Geometry: final body of the model. Coordinates: model frame, mm. Face numbers are marked on the shaded views. A direction names the side the tool comes from. Coordinates: 2 decimals unless noted, no trailing zeros. Order: outer loops, then holes, each group sorted by start corner. A loop starts at its lowest first (then second) coordinate and runs counter-clockwise, first axis right, second up. Notation, with made-up numbers: M 19.25,13 L 35.25,13 A19 ccw 35.25,47 Z; hole C 86.5,88.5 d8. An arc over 180 degrees is marked long. Write item = value, one per line.
from build123d import *

# Parameters (mm, degrees)
SKETCH1_W             = 25
SKETCH1_H             = 60
BOSS_EXTRUDE1_DEPTH   = 5
SKETCH8_W             = 5
SKETCH8_H             = 60
BOSS_EXTRUDE2_DEPTH   = 80
SKETCH9_R             = 2.1
SKETCH9_W             = 20
SKETCH9_H             = 40
CUT_EXTRUDE1_DEPTH    = 5
CUT_EXTRUDE2_REACH    = 7
FILLET1_R             = 2.5
F_3_0MM_DOWEL_HOLE1_D = 3


with BuildPart() as part:
    # Sketch1 → Boss-Extrude1 (new body)
    with BuildSketch(Plane(origin=(0, 0, 0), x_dir=(1, 0, 0), z_dir=(0, 1, 0))):
        Rectangle(SKETCH1_W, SKETCH1_H)
    extrude(amount=BOSS_EXTRUDE1_DEPTH)

    # Sketch8 → Boss-Extrude2 (add)
    with BuildSketch(Plane(origin=(0, 5, 0), x_dir=(1, 0, 0), z_dir=(0, 1, 0))):
        with Locations((-10, 0)):
            Rectangle(SKETCH8_W, SKETCH8_H)
    extrude(amount=BOSS_EXTRUDE2_DEPTH)

    # Sketch9 → Cut-Extrude1 (cut)
    with BuildSketch(Plane(origin=(-7.5, 0, 0), x_dir=(0, 0, -1), z_dir=(1, 0, 0))):
        with Locations((-5.37452771, 69.75)):
            Circle(SKETCH9_R)
        with Locations((4.62547229, 69.75)):
            Circle(SKETCH9_R)
        with Locations((-5.37452771, 20.25)):
            Circle(SKETCH9_R)
        with Locations((4.62547229, 20.25)):
            Circle(SKETCH9_R)
        with Locations((0, 45)):
            Rectangle(SKETCH9_W, SKETCH9_H)
    extrude(amount=-CUT_EXTRUDE1_DEPTH, mode=Mode.SUBTRACT)

    # Sketch10 → Cut-Extrude2 (cut, up to next)
    with BuildSketch(Plane(origin=(-7.5, 0, 0), x_dir=(0, 0, -1), z_dir=(1, 0, 0)), mode=Mode.PRIVATE) as cut_extrude2_sk1:
        Polygon((-22.928932188, 85), (-30, 77.928932188), (-30, 85), align=None)
    cut_extrude2_tool1 = extrude(cut_extrude2_sk1.sketch, amount=-CUT_EXTRUDE2_REACH, mode=Mode.PRIVATE) & part.part
    add(cut_extrude2_tool1.solids().sort_by_distance((-7.5, 82.642977, 27.642977))[0], mode=Mode.SUBTRACT)
    # Sketch10 → Cut-Extrude2 (cut, up to next)
    with BuildSketch(Plane(origin=(-7.5, 0, 0), x_dir=(0, 0, -1), z_dir=(1, 0, 0)), mode=Mode.PRIVATE) as cut_extrude2_sk2:
        Polygon((22.928932188, 85), (30, 77.928932188), (30, 85), align=None)
    cut_extrude2_tool2 = extrude(cut_extrude2_sk2.sketch, amount=-CUT_EXTRUDE2_REACH, mode=Mode.PRIVATE) & part.part
    add(cut_extrude2_tool2.solids().sort_by_distance((-7.5, 82.642977, -27.642977))[0], mode=Mode.SUBTRACT)

    # Fillet1
    fillet1_edges = [part.edges().sort_by_distance(p)[0] for p in [
        (-7.5, 5, 0),
    ]]
    fillet(fillet1_edges, radius=FILLET1_R)

    # Ø3.0mm Dowel Hole1 (through all)
    with Locations(Plane(origin=(0, 5, 0), x_dir=(1, 0, 0), z_dir=(0, 1, 0))):
        with Locations((-1.15, 7.5), (-1.15, -7.5)):
            f_3_0mm_dowel_hole1 = Hole(F_3_0MM_DOWEL_HOLE1_D / 2)

    # Mirror1: Ø3.0mm Dowel Hole1 across plane
    add(f_3_0mm_dowel_hole1.mirror(Plane(origin=(3.75, 0, 0), x_dir=(0, 0, 1), z_dir=(1, 0, 0))), mode=Mode.SUBTRACT)


solid = part.part
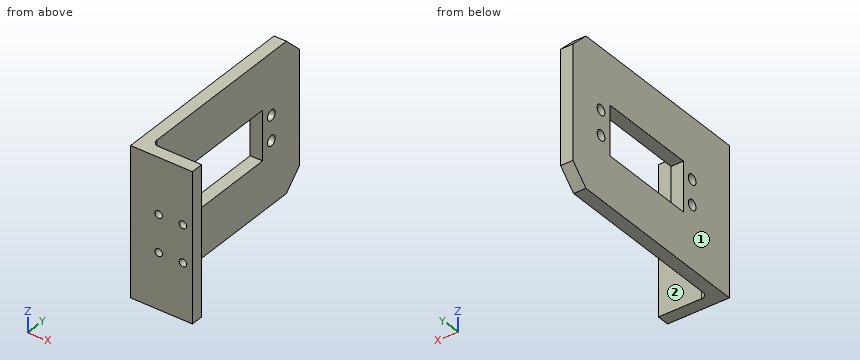
1) Section A-A, the plane x = 8.65. Return loops of the section in (y, z), and give its area (3 significant figures).
Numbers:
outline = M 0,-30 L 5,-30 L 5,-9 L 0,-9 Z; M 0,-6 L 5,-6 L 5,6 L 0,6 Z; M 0,9 L 5,9 L 5,30 L 0,30 Z
area = 270 mm²
2) Line query: L1, parallel to Y at x = -10.25, z = 7; L2, parallel to X at y = 14.5, z = -26; L3, parallel to Y at x = 9.5, z = 4.5. Output: solid intervals per line, ascending.
Numbers:
L1 = 0 to 18.92, 21.58 to 25, 65 to 68.42, 71.08 to 85
L2 = -12.5 to -7.5
L3 = 0 to 5
3) Set-up query: the marked faces 1 and 2. Return all of +Z, -Z, +X, -X, +Y, -Y with unobstructed straight access to the full face (end or side cutting, diameter ignored); none if empty.
Numbers:
face_1 = +Z, -Z, -X, +Y, -Y
face_2 = +Z, -Z, +X, +Y
4) Pin query (flat end, axial travel): pin 1 (5 mm diameter, centred on y = 69.75, z = -4.63, fed in from +X); pin 2 (6 mm diameter, centred on x = -0.5, z = -18, fed in from +Y). Return the tip coordinate at first contact, or that it passes through.
Numbers:
pin_1 = -7.5
pin_2 = 5
5) Section B-B, the plane y = 69.75. Return loops of the section in (x, z), and give its area (3 significant figures).
Numbers:
outline = M -12.5,-30 L -7.5,-30 L -7.5,-6.73 L -12.5,-6.73 Z; M -12.5,-2.53 L -7.5,-2.53 L -7.5,3.27 L -12.5,3.27 Z; M -12.5,7.47 L -7.5,7.47 L -7.5,30 L -12.5,30 Z
area = 258 mm²
6) Section C-C, the plane x = -9.25. Return loops of the section in (y, z), and give its area (3 significant figures).
Numbers:
outline = M 0,-30 L 77.93,-30 L 85,-22.93 L 85,22.93 L 77.93,30 L 0,30 Z; hole C 20.25,-4.63 d4.2; hole C 20.25,5.37 d4.2; hole M 25,-10 L 65,-10 L 65,10 L 25,10 Z; hole C 69.75,-4.63 d4.2; hole C 69.75,5.37 d4.2
area = 4,190 mm²
7) Section D-D, the plane y = 38. Return loops of the section in (x, z), and give its area (3 significant figures).
Numbers:
outline = M -12.5,-30 L -7.5,-30 L -7.5,-10 L -12.5,-10 Z; M -12.5,10 L -7.5,10 L -7.5,30 L -12.5,30 Z
area = 200 mm²
